Verification items for the finished model (mm, model axes). A direction names the side the tool comes from. Round coordinates to 2 decimals unless told otherwise and drop trailing zeros. Loops run counter-clockwise (first coordinate to the right, second up) from the corner with the lowest first, then second, coordinate; pieces in that order, holes last. Notation, with made-up numbers: (-24, 29.25) -> (-15, 29.25) arc R13 ccw to (-15, 34.25) -> close; hole circle Ø2 at (82.5, -11). An arc over 180 degrees is marked (long way). Write item = value, one per line.
```python
from build123d import *

# Parameters (mm, degrees)
PAD_DEPTH = 4


with BuildPart() as part:
    # Sketch002 → Pad (new body)
    with BuildSketch(Plane.XY):
        with BuildLine():
            Line((65, 31.5), (-10, 31.5))
            ThreePointArc((-10, 31.5), (-17.071068, 28.571068), (-20, 21.5))
            Line((-20, 21.5), (-20, 0))
            Line((-12, 0), (-20, 0))
            Line((-12, -4), (-12, 0))
            Line((18, -4), (-12, -4))
            Line((18, -4), (18, 0))
            Line((28, 0), (18, 0))
            Line((28, 0), (28, 1))
            Line((28, 1), (45, 1))
            Line((45, 1), (45, 26.5))
            Line((45, 26.5), (65, 26.5))
            Line((65, 26.5), (65, 31.5))
        make_face()
        with BuildLine():
            Line((-16, 21.5), (-16, 5.715926))
            Line((-16, 5.715926), (0, 5.715926))
            Line((0, 5.715926), (35, 5.715926))
            Line((35, 5.715926), (41, 5.715926))
            Line((41, 5.715926), (41, 27.5))
            Line((41, 27.5), (-10, 27.5))
            ThreePointArc((-10, 27.5), (-14.223161, 25.723161), (-16, 21.5))
        make_face(mode=Mode.SUBTRACT)
    extrude(amount=PAD_DEPTH)


solid = part.part
```
(1) Sectioned sample at A-A, the plane x = 27. Record the cut outline in (y, z).
Filled sheet:
outline = (0, 0) -> (5.72, 0) -> (5.72, 4) -> (0, 4) -> close; (27.5, 0) -> (31.5, 0) -> (31.5, 4) -> (27.5, 4) -> close
(2) Material ranges on probe 1 along X at (y, z) = (18, 3.15); probe 2 along Y at (x, z) = (-9.5, 0.65); probe 3 along X at (y, z) = (5.5, 2), recorded low to high. Write a range as from..to.
Filled sheet:
probe_1 = -20..-16, 41..45
probe_2 = -4..5.72, 27.5..31.5
probe_3 = -20..45
(3) Go/stop test with flat-tipped pins: pin 1 Ø0.5 at (y, z) = (0.5, 2) entering from +X; pin 2 Ø1.2 at (x, z) = (-17.5, 3) entering from -Y. Record where each tip stops, or that it passes through.
Filled sheet:
pin_1 = 28
pin_2 = 0
(4) Sectioned sample at C-C, the plane z = 2.6. Record the cut outline in (x, y), and give its area (3 significant figures).
Filled sheet:
outline = (-20, 0) -> (-12, 0) -> (-12, -4) -> (18, -4) -> (18, 0) -> (28, 0) -> (28, 1) -> (45, 1) -> (45, 26.5) -> (65, 26.5) -> (65, 31.5) -> (-10, 31.5) arc R10 ccw to (-20, 21.5) -> close; hole (-16, 5.72) -> (41, 5.72) -> (41, 27.5) -> (-10, 27.5) arc R6.07 ccw to (-16, 21.5) -> close
area = 995 mm2
(5) Sectioned sample at D-D, the plane x = 57. Record the cut outline in (y, z).
Filled sheet:
outline = (26.5, 0) -> (31.5, 0) -> (31.5, 4) -> (26.5, 4) -> close
(6) Sectioned sample at B-B, the plane y = 15. Record the cut outline in (x, z), and give its area (3 significant figures).
Filled sheet:
outline = (-20, 0) -> (-16, 0) -> (-16, 4) -> (-20, 4) -> close; (41, 0) -> (45, 0) -> (45, 4) -> (41, 4) -> close
area = 32.0 mm2
(7) Draft check along Y on faces 6 (the face through (-20, 11, 2)), 7 (the face through (28, 31.5, 2)), 8 (the face through (-14.176, 25.769, 1.972)), 9 (the face through (16, 27.5, 2)). Enter one of: released by +Y, released by -Y, zero draft, split by the parting line, or undercut.
Filled sheet:
face_6 = zero draft
face_7 = released by +Y
face_8 = undercut
face_9 = undercut
(8) Set-up check for faces 1 (the face through (-16, 0, 2)), 2 (the face through (23, 0, 2)), 3 (the face through (3, -4, 2)), 4 (the face through (41, 16, 2)), 5 (the face through (19, 5, 4)): record each of +Z, -Z, +X, -X, +Y, -Y from which the full face is reachable in a straight line by a thin tool's end or side.
Filled sheet:
face_1 = +Z, -Z, -X, -Y
face_2 = +Z, -Z, +X, -Y
face_3 = +Z, -Z, +X, -X, -Y
face_4 = +Z, -Z
face_5 = +Z, +X, -X, +Y, -Y
